Check sheet for the modelled part. Datum: model origin and axes. Units: mm. Give positions to 0.01 mm unless a question says otherwise; leave off trailing zeros. Write each loop counter-clockwise with the first axis right and the second up, starting at its lowest first coordinate (ties: lowest second). Pieces come first, ordered by that corner, then holes. Notation, with made-up numbers: (69.5, 76.5) -> (80.5, 76.5) arc R22 cw to (80.5, 103.5) -> close; hole circle Ø8 at (85, 35.25). An arc over 180 degrees is marked (long way). Use a Markdown table: item, result. Add a question column.
1. Scan lines: probe 1 along X at (y, z) = (2.35, 42.5); probe 2 along Z at (x, y) = (41.5, 3.15); probe 3 along Z at (x, y) = (-19, 4.45). Record each from-to range of solid material in increasing order. Write a range as [from, to].
2. Cross-section at B-B (x = 45). Enter the section's corners in (y, z).
3. Gauge pin test, flat ends, axial feed: P1, Ø3, axis at y = 3, z = -36, coming from the -X side; P2, Ø1, axis at x = -32.5, y = 1.5, coming from the +Z side. Record the tip position at first contact, or that the pin passes through.
4. Cross-section at C-C (z = -42.5). Enter the section's corners in (x, y), then the cut area to 3 significant figures.
5. Cross-section at A-A (y = 1.15). Enter the section's corners in (x, z).
6. Cross-section at D-D (z = -17). Enter the section's corners in (x, y).
from build123d import *

# Parameters (mm, degrees)
BOSS_EXTRU_1_DEPTH = 5
D_GAGEMENT_M31_D   = 3.6


with BuildPart() as part:
    # Esquisse1 → Boss.-Extru.1 (new body)
    with BuildSketch(Plane(origin=(0, 0, 0), x_dir=(1, 0, 0), z_dir=(0, 1, 0))):
        with BuildLine():
            Line((-47.574838249, 39.773700678), (-38.823115476, 31.508184726))
            ThreePointArc((-38.823115476, 31.508184726), (-50, 0), (-38.823115476, -31.508184726))
            Line((-38.823115476, -31.508184726), (-47.574838249, -39.773700678))
            ThreePointArc((-47.574838249, -39.773700678), (-47.726299322, -45.074838249), (-42.425161751, -45.226299322))
            Line((-42.425161751, -45.226299322), (-33.673438979, -36.96078337))
            ThreePointArc((-33.673438979, -36.96078337), (0, -50), (33.673438979, -36.96078337))
            Line((33.673438979, -36.96078337), (42.425161751, -45.226299322))
            ThreePointArc((42.425161751, -45.226299322), (47.726299322, -45.074838249), (47.574838249, -39.773700678))
            Line((47.574838249, -39.773700678), (38.823115476, -31.508184726))
            ThreePointArc((38.823115476, -31.508184726), (50, 0), (38.823115476, 31.508184726))
            Line((38.823115476, 31.508184726), (47.574838249, 39.773700678))
            ThreePointArc((47.574838249, 39.773700678), (47.726299322, 45.074838249), (42.425161751, 45.226299322))
            Line((42.425161751, 45.226299322), (33.673438979, 36.96078337))
            ThreePointArc((33.673438979, 36.96078337), (0, 50), (-33.673438979, 36.96078337))
            Line((-33.673438979, 36.96078337), (-42.425161751, 45.226299322))
            ThreePointArc((-42.425161751, 45.226299322), (-47.726299322, 45.074838249), (-47.574838249, 39.773700678))
        make_face()
    extrude(amount=BOSS_EXTRU_1_DEPTH)

    # Dégagement M31 (through all)
    with Locations(Plane(origin=(-45, 5, 42.5), x_dir=(0, 0, 1), z_dir=(0, 1, 0))):
        with Locations((0, 0), (-85, 0), (-85, 90), (0, 90)):
            Hole(D_GAGEMENT_M31_D / 2)


solid = part.part
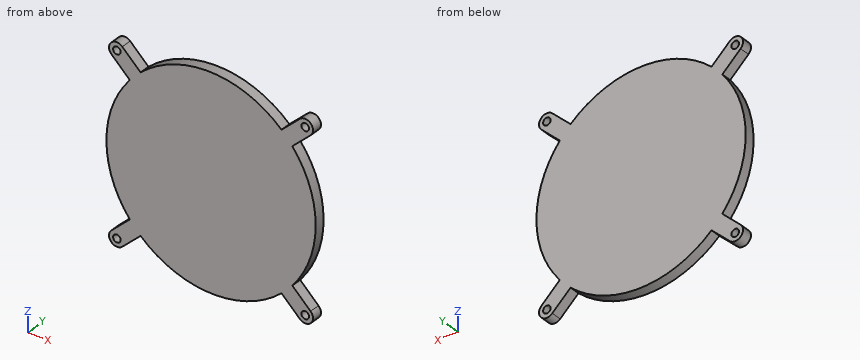
Worked answers:
| question | item | result |
|---|---|---|
| 1 | probe 1 | x = [-48.75, -46.8], [-43.2, -39.54], [-26.34, 26.34], [39.54, 43.2], [46.8, 48.75] |
| 1 | probe 2 | z = [-44.35, -34.04], [-27.89, 27.89], [34.04, 44.35] |
| 1 | probe 3 | z = [-46.25, 46.25] |
| 2 | outline | (0, -46.25) -> (5, -46.25) -> (5, -44.3) -> (0, -44.3) -> close; (0, -40.7) -> (5, -40.7) -> (5, -37.34) -> (0, -37.34) -> close; (0, -21.79) -> (5, -21.79) -> (5, 21.79) -> (0, 21.79) -> close; (0, 37.34) -> (5, 37.34) -> (5, 40.7) -> (0, 40.7) -> close; (0, 44.3) -> (5, 44.3) -> (5, 46.25) -> (0, 46.25) -> close |
| 3 | P1 | stops at x = -45.17 |
| 3 | P2 | stops at z = 38.42 |
| 4 | outline | (-48.75, 0) -> (-46.8, 0) -> (-46.8, 5) -> (-48.75, 5) -> close; (-43.2, 0) -> (-39.54, 0) -> (-39.54, 5) -> (-43.2, 5) -> close; (-26.34, 0) -> (26.34, 0) -> (26.34, 5) -> (-26.34, 5) -> close; (39.54, 0) -> (43.2, 0) -> (43.2, 5) -> (39.54, 5) -> close; (46.8, 0) -> (48.75, 0) -> (48.75, 5) -> (46.8, 5) -> close |
| 4 | area | 320 mm² |
| 5 | outline | (-47.57, -39.77) arc R3.75 ccw to (-42.43, -45.23) -> (-33.67, -36.96) arc R50 ccw to (33.67, -36.96) -> (42.43, -45.23) arc R3.75 ccw to (47.57, -39.77) -> (38.82, -31.51) arc R50 ccw to (38.82, 31.51) -> (47.57, 39.77) arc R3.75 ccw to (42.43, 45.23) -> (33.67, 36.96) arc R50 ccw to (-33.67, 36.96) -> (-42.43, 45.23) arc R3.75 ccw to (-47.57, 39.77) -> (-38.82, 31.51) arc R50 ccw to (-38.82, -31.51) -> close; hole circle Ø3.6 at (-45, -42.5); hole circle Ø3.6 at (-45, 42.5); hole circle Ø3.6 at (45, -42.5); hole circle Ø3.6 at (45, 42.5) |
| 6 | outline | (-47.02, 0) -> (47.02, 0) -> (47.02, 5) -> (-47.02, 5) -> close |
